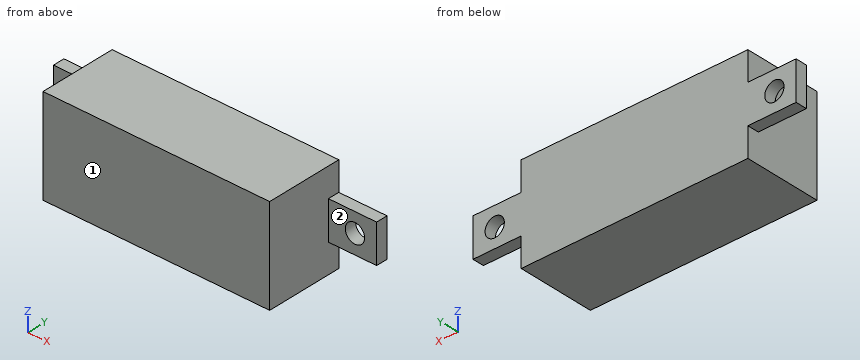
```python
from build123d import *

# Parameters (mm, degrees)
SKETCH1_W           = 23.5
SKETCH1_H           = 10
BOSS_EXTRUDE1_DEPTH = 8
SKETCH2_W           = 10
SKETCH2_H           = 4
SKETCH2_R           = 1
BOSS_EXTRUDE2_DEPTH = 1.2


with BuildPart() as part:
    # Sketch1 → Boss-Extrude1 (new body)
    with BuildSketch(Plane(origin=(0, 0, 0), x_dir=(1, 0, 0), z_dir=(0, 1, 0))):
        Rectangle(SKETCH1_W, SKETCH1_H)
    extrude(amount=BOSS_EXTRUDE1_DEPTH)

    # Sketch2 → Boss-Extrude2 (add)
    with BuildSketch(Plane(origin=(0, 8, 0), x_dir=(1, 0, 0), z_dir=(0, 1, 0))):
        with Locations((11.75, 0)):
            Rectangle(SKETCH2_W, SKETCH2_H)
        with Locations((14.5, 0)):
            Circle(SKETCH2_R, mode=Mode.SUBTRACT)
        with Locations((-11.75, 0)):
            Rectangle(SKETCH2_W, SKETCH2_H)
        with Locations((-14.5, 0)):
            Circle(SKETCH2_R, mode=Mode.SUBTRACT)
    extrude(amount=-BOSS_EXTRUDE2_DEPTH)


solid = part.part
```
The listing builds one solid part. Answer for the finished solid, in the listing's coordinates (mm). Face numbers are marked on the shaded views. A direction names the side the tool comes from. Give positions to 0.01 mm unless a question says otherwise; leave off trailing zeros. Order: outer loops, then holes, each group sorted by start corner. A loop starts at its lowest first (then second) coordinate and runs counter-clockwise, first axis right, second up. Notation, with made-up numbers: (-37, -24.75) -> (-3, -24.75) arc R9 cw to (-3, -14.75) -> close; hole circle Ø4 at (-20, 36.25). An arc over 180 degrees is marked (long way). Answer as CSV lines item,"result". Start each with the question number.
Q1. A cutting plane is placed at B-B (x = 14.5). Determine the outline of the cut face in (y, z), then the cut area to 3 significant figures.
Q2. A cutting plane is placed at C-C (y = 1). Determine the outline of the cut face in (x, z), then the cut area to 3 significant figures.
Q3. Which of the six approach directions +Z, -Z, +X, -X, +Y, -Y give full straight-line access (tool end or side, diameter ignored) to the marked faces 1 and 2?
Q4. Given pin 1 (3 mm diameter, centred on x = 13.5, z = 1, fed in from -Y); pin 2 (1 mm diameter, centred on x = -13.5, y = 7.5, fed in from -Z); pin 3 (1 mm diameter, centred on y = 2.5, z = -1, fed in from +X), each flat-ended and moving along its own axis, determine where each tip first touches the part or whether it passes through.
Q5. A cutting plane is placed at D-D (z = 3.25). Determine the outline of the cut face in (x, y).
Q6. A cutting plane is placed at A-A (z = 0). Determine the outline of the cut face in (x, y).
Q7. Find the intervals of material crossed by L1, parallel to X at y = 7.1, z = 0; L2, parallel to X at y = 7, z = -0.5; L3, parallel to Z at x = -14.5, y = 7.4, in increasing order.
Results found:
1,outline,"(6.8, -2) -> (8, -2) -> (8, -1) -> (6.8, -1) -> close; (6.8, 1) -> (8, 1) -> (8, 2) -> (6.8, 2) -> close"
1,area,"2.40 mm2"
2,outline,"(-11.75, -5) -> (11.75, -5) -> (11.75, 5) -> (-11.75, 5) -> close"
2,area,"235 mm2"
3,face 1,"+Z, -Z, +X, -X, -Y"
3,face 2,"+Z, -Z, +X, -Y"
4,pin 1,"y = 6.8"
4,pin 2,"z = -2"
4,pin 3,"x = 11.75"
5,outline,"(-11.75, 0) -> (11.75, 0) -> (11.75, 8) -> (-11.75, 8) -> close"
6,outline,"(-16.75, 6.8) -> (-15.5, 6.8) -> (-15.5, 8) -> (-16.75, 8) -> close; (-13.5, 6.8) -> (-11.75, 6.8) -> (-11.75, 0) -> (11.75, 0) -> (11.75, 6.8) -> (13.5, 6.8) -> (13.5, 8) -> (-13.5, 8) -> close; (15.5, 6.8) -> (16.75, 6.8) -> (16.75, 8) -> (15.5, 8) -> close"
7,L1,"-16.75 to -15.5, -13.5 to 13.5, 15.5 to 16.75"
7,L2,"-16.75 to -15.37, -13.63 to 13.63, 15.37 to 16.75"
7,L3,"-2 to -1, 1 to 2"
